```python
from build123d import *

# Parameters (mm, degrees)
F0_W     = 20
F0_H     = 20
F0_R     = 1.75
F1_DEPTH = 2
F0_R_2   = 2
F2_DEPTH = 6


# Not quite as in the source:
# - a feature names something its author has since deleted; it is built from what else it names


with BuildPart() as f1:
    # F0 (on Front) → F1 (new body)
    with BuildSketch(Plane.XZ):
        Polygon((-29.00025, 5.7325412996), (-29.00025, 25.7325412996), (-9.00025, 25.7325412996), (-9.00025, 5.7325412996), (-7.00025, 5.7325412996), (-7.00025, 14.311070554), (-7.00025, 22.311070554), (-7.00025, 28.4722108253), (-31.00025, 28.4722108253), (-31.00025, 22.311070554), (-31.00025, 14.311070554), (-31.00025, 5.7325412996), align=None)
        with Locations((-19.00025, 15.7325412996)):
            Rectangle(F0_W, F0_H)
        with Locations((-19.00025, 15.7325412996)):
            Circle(F0_R, mode=Mode.SUBTRACT)
        with Locations((-19.00025, 15.7325412996)):
            Circle(F0_R)
    extrude(amount=F1_DEPTH)

    # F0 (on Front) → F2 (join)
    with BuildSketch(Plane.XZ):
        Polygon((-29.00025, 5.7325412996), (-29.00025, 25.7325412996), (-9.00025, 25.7325412996), (-9.00025, 5.7325412996), (-7.00025, 5.7325412996), (-7.00025, 14.311070554), (-7.00025, 22.311070554), (-7.00025, 28.4722108253), (-31.00025, 28.4722108253), (-31.00025, 22.311070554), (-31.00025, 14.311070554), (-31.00025, 5.7325412996), align=None)
        with BuildLine():
            Line((-7.00025, 22.311070554), (-7.00025, 14.311070554))
            Line((-7.00025, 14.311070554), (-4, 14.311070554))
            ThreePointArc((-4, 14.311070554), (-1.1715728753, 15.4826434292), (0, 18.311070554))
            ThreePointArc((0, 18.311070554), (-1.1715728753, 21.1394976787), (-4, 22.311070554))
            Line((-4, 22.311070554), (-7.00025, 22.311070554))
        make_face()
        with Locations((-4, 18.311070554)):
            Circle(F0_R_2, mode=Mode.SUBTRACT)
        with Locations((-19.00025, 15.7325412996)):
            Circle(F0_R)
        with BuildLine():
            Line((-34.1055206901, 14.311070554), (-31.00025, 14.311070554))
            Line((-31.00025, 14.311070554), (-31.00025, 22.311070554))
            Line((-31.00025, 22.311070554), (-34.1055206901, 22.311070554))
            ThreePointArc((-34.1055206901, 22.311070554), (-38.1055206901, 18.311070554), (-34.1055206901, 14.311070554))
        make_face()
        with Locations((-34, 18.311070554)):
            Circle(F0_R_2, mode=Mode.SUBTRACT)
    extrude(amount=-F2_DEPTH)


solid = f1.part
```
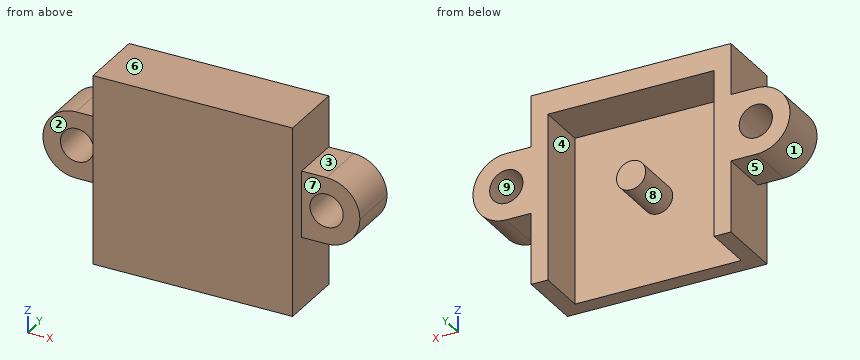
The model under review builds one solid part; all positions refer to its coordinate system, in mm. Face numbers are marked on the shaded views. A direction names the side the tool comes from. Round coordinates to 2 decimals unless told otherwise and drop trailing zeros. Order: outer loops, then holes, each group sorted by start corner. A loop starts at its lowest first (then second) coordinate and runs counter-clockwise, first axis right, second up. Notation, with made-up numbers: M 55.25,-12 L 73.25,-12 A7 ccw 73.25,1 Z; hole C 46,-14 d1. An arc over 180 degrees is marked long. Use a Markdown table: item, result.
1) Consider section D-D (z = 26.25). Write out the cut boundary in (x, y), then the cut area to 3 significant figures.
Report:
| item | result |
|---|---|
| outline | M -31,-2 L -7,-2 L -7,6 L -31,6 Z |
| area | 192 mm^2 |
2) Draft analysis for pull direction Z (two halves, no side actions). For the marked faces 6, 7, 8 and 9, state which applies: released by +Z, released by -Z, zero draft, split by the parting line, or undercut.
Report:
| item | result |
|---|---|
| face 6 | released by +Z |
| face 7 | zero draft |
| face 8 | undercut |
| face 9 | undercut |
3) Consider section C-C (x = -25). Write out the cut boundary in (y, z), then the cut area to 3 significant figures.
Report:
| item | result |
|---|---|
| outline | M -2,5.73 L 0,5.73 L 0,25.73 L 6,25.73 L 6,28.47 L -2,28.47 Z |
| area | 61.9 mm^2 |
4) Wall thickness on line 1 along X through (y, z) = (1, 7.25); line 2 along X through (y, z) = (2.25, 17); line 3 along X through (y, z) = (5.5, 17.75): over which ranges is each line inside the solid? List them lowest first. Write a range as [from, to].
Report:
| item | result |
|---|---|
| line 1 | [-31, -29], [-9, -7] |
| line 2 | [-37.88, -35.51], [-32.49, -29], [-20.21, -17.79], [-9, -5.51], [-2.49, -0.22] |
| line 3 | [-38.07, -35.92], [-32.08, -29], [-9, -5.92], [-2.08, -0.04] |
5) Insertion check: pin 1 (1.5 mm diameter, centred on x = -6, y = 2, fed in from -Z); pin 2 (1.8 mm diameter, centred on x = -19, y = 4, fed in from -Z); pin 3 (2.5 mm diameter, centred on x = -33, y = 2, fed in from +Z). Each pin has a flat end and moves straight along its axis. Give the tip position at first contact, or say it passes through.
Report:
| item | result |
|---|---|
| pin 1 | z = 14.31 |
| pin 2 | z = 13.98 |
| pin 3 | z = 22.31 |
6) Tool access review of the marked faces 1, 2, 3, 4 and 5: name each direction out of +Z, -Z, +X, -X, +Y, -Y from which nothing blocks a thin tool from reaching the whole face with its end or side.
Report:
| item | result |
|---|---|
| face 1 | -X, +Y, -Y |
| face 2 | +Z, -Z, -X, -Y |
| face 3 | +Z, +X, +Y, -Y |
| face 4 | -Z, +Y |
| face 5 | -Z, -X, +Y, -Y |
7) Consider section B-B (z = 12.5). Write out the cut boundary in (x, y), then the cut area to 3 significant figures.
Report:
| item | result |
|---|---|
| outline | M -31,-2 L -7,-2 L -7,6 L -9,6 L -9,0 L -29,0 L -29,6 L -31,6 Z |
| area | 72.0 mm^2 |
8) Consider section A-A (y = 2). Write out the cut boundary in (x, z).
Report:
| item | result |
|---|---|
| outline | M -34.11,14.31 L -31,14.31 L -31,5.73 L -29,5.73 L -29,25.73 L -9,25.73 L -9,5.73 L -7,5.73 L -7,14.31 L -4,14.31 A4 ccw -4,22.31 L -7,22.31 L -7,28.47 L -31,28.47 L -31,22.31 L -34.11,22.31 A4 ccw Z; C -19,15.73 d3.5; hole C -34,18.31 d4; hole C -4,18.31 d4 |
